For this review, take the finished solid that the model builds, in its own axes (mm). A direction names the side the tool comes from. Coordinates: 2 decimals unless noted, no trailing zeros. Loops run counter-clockwise (first coordinate to the right, second up) from the corner with the lowest first, then second, coordinate; pieces in that order, holes last. Notation, with made-up numbers: M 40,83 L 44,83 A26 cw 44,99 Z; hole C 46.25,10 d3. An arc over 180 degrees is marked long. Answer as a JSON object with one key per item and string values. Group by question number.
Item 1: Tool access review of faces 1 (the face through (17.5, 1.4, 1.4)), 2 (the face through (26, 6.829, 0)), 3 (the face through (3.805, -17.741, 0.233)), 4 (the face through (8, 8, -12)), 5 (the face through (2.71, 2.82, 9.61)): name each direction out of +Z, -Z, +X, -X, +Y, -Y from which nothing blocks a thin tool from reaching the whole face with its end or side.
Item 2: Mouldability with a two-part tool opening along Y and no side actions: class faces 6 (the face through (7, 4.45, 0)), 7 (the face through (30.571, -23.272, -0.233)), 8 (the face through (4.71, 12.44, -6.08)), 9 (the face through (17.085, 9.294, 0.233)) as +Y half, -Y half, draft (parallel to the pull), parting line (faces both ways), or undercut.
Item 3: Wall thickness on L1, parallel to Z at x = 12.5, y = -5; L2, parallel to Z at x = 5, y = -2; L3, parallel to X at y = -19, z = 4: over which ranges is each line inside the solid? List them lowest first. Write a range as from..to.
Item 4: Add section A-A (y = 7.95). State the section outline as (x, z) points.
Item 5: Add section B-B (z = 14.5). State the section outline as (x, y) points, then the cut area to 3 significant figures.
Item 6: Insertion check: pin 1 (2 mm diameter, centred on x = 4.5, y = 8, fed in from +Z); pin 2 (2.5 mm diameter, centred on y = 0, z = 1.5, fed in from +X); pin 3 (13.5 mm diameter, centred on y = 19.5, z = 6.5, fed in from +X); pin 4 (13.5 mm diameter, centred on x = 25, z = -6, fed in from +Y). Each pin has a flat end and moves straight along its axis. Give the tip position at first contact, or say it passes through.
from build123d import *

# Parameters (mm, degrees)
SKETCH1_W               = 33.3
SKETCH1_H               = 48.3
BOSS_EXTRUDE1_DEPTH     = 9.55
CUT_EXTRUDE1_DEPTH      = 5.5
SKETCH3_W               = 5.65
SKETCH3_H               = 13.7
CUT_EXTRUDE2_DEPTH      = 5
SKETCH5_W               = 33.3
SKETCH5_H               = 48.3
BOSS_EXTRUDE3_DEPTH     = 22.5
SKETCH6_R               = 4.025
CUT_EXTRUDE3_DEPTH      = 12
SKETCH7_R               = 4.75
CUT_EXTRUDE4_DEPTH      = 14.55
CUT_EXTRUDE6_DEPTH      = 46.909857329
CUT_EXTRUDE6_DEPTH_BACK = 46.909857329
SKETCH27_R              = 2
SKETCH30_R              = 4
SKETCH31_R              = 5
CHAMFER1_SIZE           = 13
CHAMFER1_SIZE2          = 7.505553499
CHAMFER2_SIZE           = 10
CHAMFER2_SIZE2          = 17.320508076
CHAMFER3_SIZE           = 1.732050808
CHAMFER3_SIZE_2         = 3
CROQUIS2_W              = 17.5
CROQUIS2_H              = 17.320508076
CORTAR_EXTRUIR1_DEPTH   = 48
CHAMFER4_SIZE           = 5


with BuildPart() as part:
    # Sketch1 → Boss-Extrude1 (new body)
    with BuildSketch(Plane(origin=(0, 0, 0), x_dir=(0, 0, -1), z_dir=(1, 0, 0))):
        Rectangle(SKETCH1_W, SKETCH1_H)
    extrude(amount=BOSS_EXTRUDE1_DEPTH)

    # Sketch2 → Cut-Extrude1 (cut)
    # profile 1 of 2: a face of its own
    with BuildSketch(Plane.ZY):
        Polygon((-5.5, 13.039115125), (-5.5, 20.15), (4.5, 20.15), (6.65, 20.15), (6.65, 5.993768204), (12.65, -0.443622572), (12.65, -9.1), (12.65, -10.95), (-12.65, -10.95), (-12.65, -9.1), (-12.65, -0.443622572), (-6.65, 5.993768204), (-6.65, 11.855899168), align=None)
        Polygon((4.5, 19.15), (5.65, 19.15), (5.65, 5.6), (11.65, -0.837390776), (11.65, -9.1), (11.65, -9.95), (-11.65, -9.95), (-11.65, -9.1), (-11.65, -0.837390776), (-5.65, 5.6), (-5.65, 11.45), (-4.5, 12.633215957), (-4.5, 19.15), align=None, mode=Mode.SUBTRACT)
    # profile 2 of 2: a face of its own
    with BuildSketch(Plane.ZY):
        Polygon((5.65, 19.15), (5.65, 5.6), (11.65, -0.837390776), (11.65, -9.1), (11.65, -9.95), (-11.65, -9.95), (-11.65, -9.1), (-11.65, -0.837390776), (-5.65, 5.6), (-5.65, 11.45), (-4.5, 12.633215957), (-4.5, 19.15), (4.5, 19.15), align=None)
    extrude(amount=-CUT_EXTRUDE1_DEPTH, mode=Mode.SUBTRACT)

    # Sketch3 → Cut-Extrude2 (cut)
    # profile 1 of 3: a face of its own
    with BuildSketch(Plane.ZY.offset(-5.5)):
        Polygon((-6.65, 4.45), (6.65, 4.45), (6.65, 20.15), (-5.5, 20.15), (-5.5, 13.039115125), (-6.65, 11.855899168), align=None)
        Polygon((5.65, 5.45), (5.65, 19.15), (-4.5, 19.15), (-4.5, 12.633215957), (-5.65, 11.45), (-5.65, 5.45), align=None, mode=Mode.SUBTRACT)
    # profile 2 of 3: a face of its own
    with BuildSketch(Plane.ZY.offset(-5.5)):
        Polygon((0, 5.45), (0, 19.15), (-4.5, 19.15), (-4.5, 12.633215957), (-5.65, 11.45), (-5.65, 5.45), align=None)
    # profile 3 of 3: a face of its own
    with BuildSketch(Plane.ZY.offset(-5.5)):
        with Locations((2.825, 12.3)):
            Rectangle(SKETCH3_W, SKETCH3_H)
    extrude(amount=-CUT_EXTRUDE2_DEPTH, mode=Mode.SUBTRACT)

    # Sketch5 → Boss-Extrude3 (add)
    with BuildSketch(Plane(origin=(9.55, 0, 0), x_dir=(0, 0, -1), z_dir=(1, 0, 0))):
        Rectangle(SKETCH5_W, SKETCH5_H)
    extrude(amount=BOSS_EXTRUDE3_DEPTH)

    # Sketch6 → Cut-Extrude3 (cut)
    with BuildSketch(Plane.ZY.offset(-5.5)):
        with Locations((0, -2.575)):
            Circle(SKETCH6_R)
    extrude(amount=-CUT_EXTRUDE3_DEPTH, mode=Mode.SUBTRACT)

    # Sketch7 → Cut-Extrude4 (cut)
    with BuildSketch(Plane.ZY.offset(-17.5)):
        with Locations((0, -2.575)):
            Circle(SKETCH7_R)
    extrude(amount=-CUT_EXTRUDE4_DEPTH, mode=Mode.SUBTRACT)

    # Sketch27 → Cut-Extrude6 (cut, two sides: drawn at the far end of the back side and taken through both)
    with BuildSketch(Plane(origin=(0, 0, 5.65), x_dir=(-1, 0, 0), z_dir=(0, 0, -1)).offset(-CUT_EXTRUDE6_DEPTH_BACK)):
        with Locations((-6, 7.95)):
            Circle(SKETCH27_R)
    extrude(amount=CUT_EXTRUDE6_DEPTH + CUT_EXTRUDE6_DEPTH_BACK, mode=Mode.SUBTRACT)

    # Cut-Sweep1: sweep along a path in Sketch28
    with BuildLine(Plane.XY) as cut_sweep1_path:
        Line((25.736872918, -27.79488562), (13.5, -6.6))
        Line((13.5, -6.6), (11.25, -2.702885683))
    # Sketch30 → Cut-Sweep1 (sweep, cut)
    with BuildSketch(Plane(origin=(18.469756751, -31.990557096, 0), x_dir=(0, 0, -1), z_dir=(0.500000000000001, -0.866025403784438, 0))):
        with Locations((0, 8.391342951)):
            Circle(SKETCH30_R)
    sweep(path=cut_sweep1_path.line, mode=Mode.SUBTRACT)

    # Cut-Sweep2: sweep along a path in Sketch29
    with BuildLine(Plane.XY) as cut_sweep2_path:
        Line((19.5, -16.992304845), (25.736872918, -27.79488562))
    # Sketch31 → Cut-Sweep2 (sweep, cut)
    with BuildSketch(Plane(origin=(18.469756751, -31.990557096, 0), x_dir=(0, 0, -1), z_dir=(0.500000000000001, -0.866025403784438, 0))):
        with Locations((0, 8.391342951)):
            Circle(SKETCH31_R)
    sweep(path=cut_sweep2_path.line, mode=Mode.SUBTRACT)

    # Chamfer1
    chamfer1_edges = [part.edges().sort_by_distance(p)[0] for p in [
        (0, -24.15, 0),
    ]]
    chamfer1_side = [part.faces().sort_by_distance(p)[0] for p in [
        (0, 23.563333144, 0),
    ]]
    chamfer(chamfer1_edges, length=CHAMFER1_SIZE, length2=CHAMFER1_SIZE2, reference=chamfer1_side[0])

    # Chamfer2
    chamfer2_edges = [part.edges().sort_by_distance(p)[0] for p in [
        (32.05, 24.15, 0),
    ]]
    chamfer2_side = [part.faces().sort_by_distance(p)[0] for p in [
        (16.025, 24.15, 0),
    ]]
    chamfer(chamfer2_edges, length=CHAMFER2_SIZE, length2=CHAMFER2_SIZE2, reference=chamfer2_side[0])

    # Chamfer3
    # the kernel refuses this chamfer: 3, 1.732050808 mm, written as the material it takes off along each edge
    with BuildSketch(Plane(origin=(32.05, -24.15, -24.411257264), x_dir=(0.05789386240267215, 0.9983227437537925, 0), z_dir=(0, 0, 1))) as chamfer3_piece_1:
        Polygon((CHAMFER3_SIZE * 0.998322743505, CHAMFER3_SIZE * 0.0578938623883), (-CHAMFER3_SIZE_2 * 0.0578938624027, CHAMFER3_SIZE_2 * 0.998322743754), (0, 0), align=None)
    extrude(amount=48.822514528, mode=Mode.SUBTRACT)

    # Croquis2 → Cortar-Extruir1 (cut)
    with BuildSketch(Plane.XY.offset(16.65)):
        with Locations((23.3, 15.489745962)):
            Rectangle(CROQUIS2_W, CROQUIS2_H)
    extrude(amount=-CORTAR_EXTRUIR1_DEPTH, mode=Mode.SUBTRACT)

    # Chamfer4
    chamfer4_edges = [part.edges().sort_by_distance(p)[0] for p in [
        (14.55, 6.829491924, 0),
    ]]
    chamfer(chamfer4_edges, length=CHAMFER4_SIZE)

    # Sketch33 → Cut-Loft2 section 0
    with BuildSketch(Plane.ZY):
        with BuildLine():
            Line((0, -9.95), (0, -15.45))
            Line((0, -15.45), (2.5, -15.45))
            Line((2.5, -15.45), (2.5, -9.95))
            Line((2.5, -9.95), (0, -9.95))
        make_face()
    # Sketch34 → Cut-Loft2 section 1
    with BuildSketch(Plane.ZY.offset(-5.5)):
        with BuildLine():
            Line((0, -9.95), (2.5, -9.95))
            Line((2.5, -9.95), (2.5, -10.45))
            Line((2.5, -10.45), (0, -10.45))
            Line((0, -10.45), (0, -9.95))
        make_face()
    loft(mode=Mode.SUBTRACT)


solid = part.part
From the geometry:
{
 "1": {"face 1": "+X", "face 2": "+Z, -Z, +X, +Y", "face 3": "+Z, -Z, -X, -Y", "face 4": "+Z, -Z", "face 5": "-X"},
 "2": {"face 6": "undercut", "face 7": "-Y half", "face 8": "undercut", "face 9": "+Y half"},
 "3": {"L1": "z = -16.65..-4, 4..16.65", "L2": "z = -16.65..-12.65, 12.65..16.65", "L3": "x = 4.53..17.2, 24.12..32.05"},
 "4": {"outline": "M 0,-16.65 L 4,-16.65 L 4,-6.65 L 0,-6.65 Z; M 0,6.65 L 4,6.65 L 4,16.65 L 0,16.65 Z; M 8,-16.65 L 18.43,-16.65 L 18.43,16.65 L 8,16.65 L 8,6.65 L 9.55,6.65 L 9.55,-6.65 L 8,-6.65 Z"},
 "5": {"outline": "M 0,-11.15 L 7.51,-24.15 L 29.05,-24.15 L 32.05,-22.42 L 32.05,6.83 L 19.55,6.83 L 14.55,11.83 L 14.55,24.15 L 0,24.15 Z; hole C 6,7.95 d4", "area": "1,190 mm²"},
 "6": {"pin 1": "stops at z = 16.65", "pin 2": "stops at x = 17.5", "pin 3": "stops at x = 14.55", "pin 4": "stops at y = 8.13"}
}
